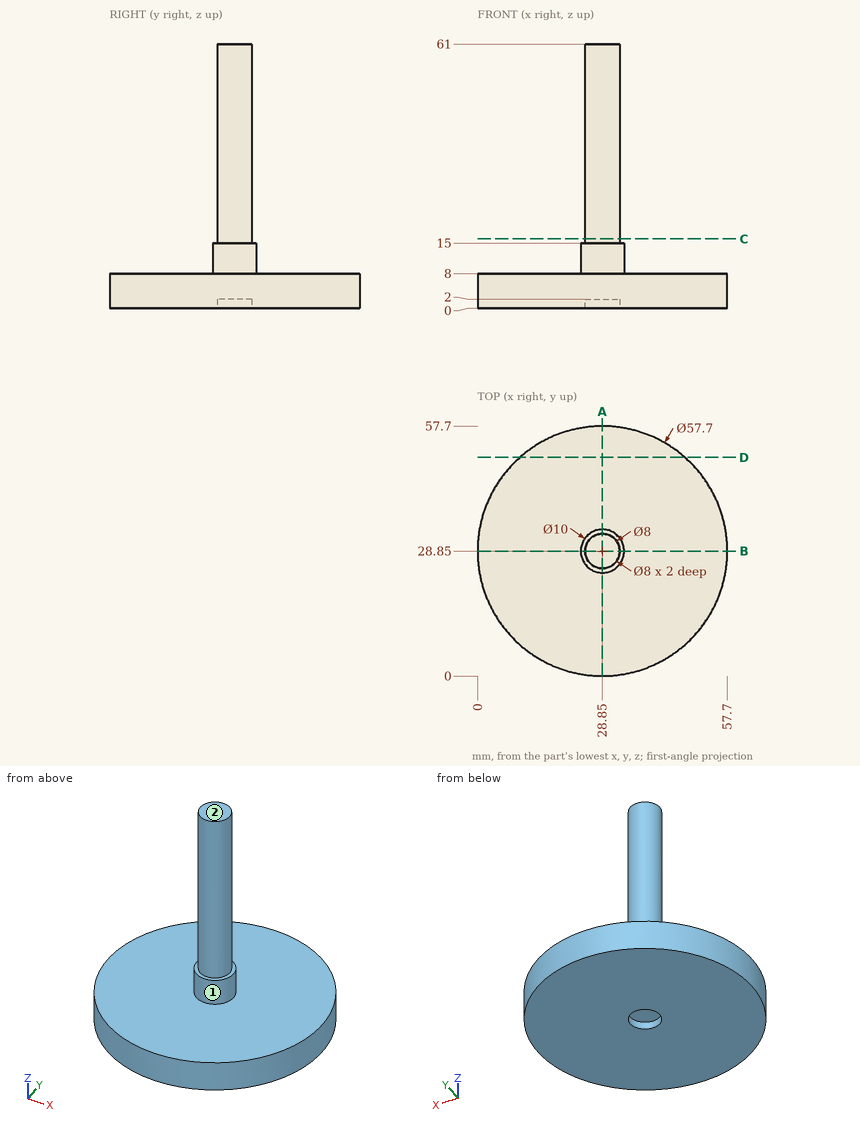
The drawing under review shows one solid part. Ordinate dimensions are in mm from its lowest x, y, z. A direction names the side the tool comes from. Round coordinates to 2 decimals unless told otherwise and drop trailing zeros. Loops run counter-clockwise (first coordinate to the right, second up) from the corner with the lowest first, then second, coordinate; pieces in that order, holes last. Notation, with made-up numbers: (9, 25) - (61, 25) arc R17 cw to (61, 51) - close; hole circle Ø11 at (-15.5, 11.5). An arc over 180 degrees is marked (long way). One line per item, written item: value. Start each with the question number.
1) Insertion check: pin 1 Ø7 at (x, y) = (28.85, 28.85) entering from -Z; pin 2 Ø3 at (x, z) = (27, 41.5) entering from -Y; pin 3 Ø4 at (x, y) = (47, 50.5) entering from -Z; pin 4 Ø2 at (y, z) = (34, 12.5) entering from -X. Each pin has a flat end and moves straight along its axis. Give the tip position at first contact, or say it passes through.
2) Consider section D-D on y = 50.5. Give the boundary of the cut face in (x, z).
3) Consider section A-A on x = 28.85. Give the boundary of the cut face in (y, z), then the cut area to 3 significant figures.
4) To check wall thickness, follow L1, parallel to Y at x = 28.85, z = 0.75; L2, parallel to Z at x = 4, y = 41; L3, parallel to X at y = 28, z = 1. State the ranges of each line that lie inside material, in increasing order. Write a range as from..to.
5) Consider section C-C on z = 16. Give the boundary of the cut face in (x, y).
6) For the marked faces 1 and 2, list the 3-axis set-ups (+Z, -Z, +X, -X, +Y, -Y) from which the entire face can be reached by the end or side of a thin tool; tool diameter is ignored.
Reported:
1. pin 1: stops at z = 2
1. pin 2: stops at y = 24.87
1. pin 3: stops at z = 0
1. pin 4: stops at x = 26.06
2. outline: (9.78, 0) - (47.92, 0) - (47.92, 8) - (9.78, 8) - close
3. outline: (0, 0) - (24.85, 0) - (24.85, 2) - (32.85, 2) - (32.85, 0) - (57.7, 0) - (57.7, 8) - (33.85, 8) - (33.85, 15) - (32.85, 15) - (32.85, 61) - (24.85, 61) - (24.85, 15) - (23.85, 15) - (23.85, 8) - (0, 8) - close
3. area: 884 mm^2
4. L1: y = 0..24.85, 32.85..57.7
4. L2: z = 0..8
4. L3: x = 0.01..24.94, 32.76..57.69
5. outline: circle Ø8 at (28.85, 28.85)
6. face 1: +Z
6. face 2: +Z, +X, -X, +Y, -Y
